Read the model definition and answer for the solid it produces. Units are mm, in the model's axes. A direction names the side the tool comes from. Give positions to 0.01 mm unless a question says otherwise; leave off trailing zeros. Order: outer loops, then holes, each group sorted by start corner. A loop starts at its lowest first (then second) coordinate and runs counter-clockwise, first axis right, second up. Notation, with made-up numbers: M 86,1.25 L 97,1.25 A11 cw 97,13.25 Z; hole C 44.25,30 d1. An arc over 180 degrees is marked long. One line per item, written item: value. Start each with the question number.
from build123d import *

# Parameters (mm, degrees)
SKETCH9_R                       = 9
SKETCH9_R_2                     = 8
BOSS_EXTRUDE1_DEPTH             = 20
SKETCH10_W                      = 4.934959926
SKETCH10_H                      = 0.2
CUT_EXTRUDE1_DEPTH              = 20
SKETCH11_R                      = 6
BOSS_EXTRUDE2_DEPTH             = 100
BOSS_EXTRUDE2_DIRECTION_2_REACH = 23.728
SKETCH12_R                      = 6
BOSS_EXTRUDE3_DEPTH             = 100
BOSS_EXTRUDE3_DIRECTION_2_REACH = 74.864
SKETCH14_R                      = 12.5
CUT_EXTRUDE3_DEPTH              = 82.317279836
CUT_EXTRUDE3_DEPTH_BACK         = 82.317279836


with BuildPart() as part:
    # Sketch9 → Boss-Extrude1 (new body)
    with BuildSketch(Plane.XY):
        Circle(SKETCH9_R)
        Circle(SKETCH9_R_2, mode=Mode.SUBTRACT)
    extrude(amount=BOSS_EXTRUDE1_DEPTH)

    # Sketch10 → Cut-Extrude1 (cut)
    with BuildSketch(Plane.XY.offset(20)):
        with Locations((8, 0)):
            Rectangle(SKETCH10_W, SKETCH10_H)
    extrude(amount=-CUT_EXTRUDE1_DEPTH, mode=Mode.SUBTRACT)

    # Sketch11 → Boss-Extrude2 (add)
    with BuildSketch(Plane(origin=(-6.363961031, 6.363961031, 0), x_dir=(0, 0, -1), z_dir=(-0.707106781, 0.707106781, 0))):
        with Locations((-10, 0)):
            Circle(SKETCH11_R)
    extrude(amount=BOSS_EXTRUDE2_DEPTH)

    # Sketch11 → Boss-Extrude2 direction 2 (add, up to next)
    with BuildSketch(Plane(origin=(-6.363961031, 6.363961031, 0), x_dir=(0, 0, -1), z_dir=(-0.707106781, 0.707106781, 0)), mode=Mode.PRIVATE) as boss_extrude2_direction_2_sk1:
        with Locations((-10, 0)):
            Circle(SKETCH11_R)
    boss_extrude2_direction_2_tool1 = extrude(boss_extrude2_direction_2_sk1.sketch, amount=-BOSS_EXTRUDE2_DIRECTION_2_REACH, mode=Mode.PRIVATE) - part.part
    add(boss_extrude2_direction_2_tool1.solids().sort_by_distance((-6.363961, 6.363961, 10))[0])
    add(boss_extrude2_direction_2_tool1.solids().sort_by_distance((-6.363961, 6.363961, 10))[1])

    # Sketch12 → Boss-Extrude3 (add)
    with BuildSketch(Plane(origin=(6.363961031, 6.363961031, 0), x_dir=(0, 0, -1), z_dir=(0.707106781, 0.707106781, 0))):
        with Locations((-10, 0)):
            Circle(SKETCH12_R)
    extrude(amount=BOSS_EXTRUDE3_DEPTH)

    # Sketch12 → Boss-Extrude3 direction 2 (add, up to next)
    with BuildSketch(Plane(origin=(6.363961031, 6.363961031, 0), x_dir=(0, 0, -1), z_dir=(0.707106781, 0.707106781, 0)), mode=Mode.PRIVATE) as boss_extrude3_direction_2_sk1:
        with Locations((-10, 0)):
            Circle(SKETCH12_R)
    boss_extrude3_direction_2_tool1 = extrude(boss_extrude3_direction_2_sk1.sketch, amount=-BOSS_EXTRUDE3_DIRECTION_2_REACH, mode=Mode.PRIVATE) - part.part
    add(boss_extrude3_direction_2_tool1.solids().sort_by_distance((6.363961, 6.363961, 10))[0])
    add(boss_extrude3_direction_2_tool1.solids().sort_by_distance((6.363961, 6.363961, 10))[1])

    # Sketch14 → Cut-Extrude3 (cut, two sides)
    with BuildSketch(Plane(origin=(0, 0, 0), x_dir=(0, 0, -1), z_dir=(1, 0, 0))) as cut_extrude3_sk:
        with Locations((-10, 79.9)):
            Circle(SKETCH14_R)
    extrude(amount=CUT_EXTRUDE3_DEPTH, mode=Mode.SUBTRACT)
    extrude(cut_extrude3_sk.sketch, amount=-CUT_EXTRUDE3_DEPTH_BACK, mode=Mode.SUBTRACT)


solid = part.part
Q1. Determine the mould class of faces 1 (the cylindrical face through (-8, 0, 10)), 2 (the cylindrical face through (67.3, 67.4, 10.1)) for opening direction X: released by +X, released by -X, zero draft, split by the parting line, or undercut.
Q2. Consider probe 1 along Y at (x, z) = (0, 13.25); probe 2 along X at (y, z) = (-1, 14); probe 3 along X at (y, z) = (0, 12.75). Determine where each line is inside the solid, lowest interval first.
Q3. Find section A-A, the plane z = 8.5. Give the vertices of the cut face in (x, y).
Q4. A tool of negligible diameter and unlimited length cuts with its end or side. For faces 3 (the cylindrical face through (-67.3, 67.4, 10.1)), 4 (the cylindrical face through (-1.993, -8.777, 9.86)), from which of +Z, -Z, +X, -X, +Y, -Y can it reach the whole face along a straight path? Write none if from no direction.
Q5. Each of these flat-tipped pins is pushed along its axis until it touches: pin 1 (8 mm diameter, centred on x = 23, z = 8, fed in from +Y); pin 2 (12 mm diameter, centred on y = 21, z = 3.5, fed in from -X); pin 3 (6 mm diameter, centred on x = 20.5, z = 14.5, fed in from +Y); pin 4 (21 mm diameter, centred on x = 0, y = 0, fed in from -Z). Where does it stop, or does it pass through?
Evaluation:
1. face 1: undercut
1. face 2: zero draft
2. probe 1: -9 to -8, 8 to 9
2. probe 2: -8.94 to -7.94, 7.94 to 8.94
2. probe 3: -9 to -8
3. outline: M -75.71,67.49 L -8.97,0.75 A9 ccw long 9,-0.1 L 8,-0.1 A8 cw long 8,0.1 L 9,0.1 A9 ccw 8.97,0.75 L 75.71,67.49 L 59.27,67.49 L 0.75,8.97 A9 ccw -0.75,8.97 L -59.27,67.49 Z
4. face 3: +X, -X, +Y
4. face 4: none
5. pin 1: y = 35.24
5. pin 2: x = -33.23
5. pin 3: y = 30.48
5. pin 4: z = 0
